Autodesk Inventor part; units mm, degrees
ref_plane "YZ Plane" through (0, 0, 0) normal (1, 0, 0) x (0, 1, 0)
ref_plane "XZ Plane" through (0, 0, 0) normal (0, 1, 0) x (-1, 0, 0)
ref_plane "XY Plane" through (0, 0, 0) normal (0, 0, 1) x (1, 0, 0)
sketch "Sketch1" plane through (0, 0, 0) normal (0, 0, 1) x (1, 0, 0)
  line L0 (-40, -28.4) -> (40, -28.4)
  line L1 (40, -28.4) -> (40, 28.4)
  line L2 (40, 28.4) -> (-40, 28.4)
  line L3 (-40, 28.4) -> (-40, -28.4)
  line L4 (-40, -28.4) -> (40, 28.4) construction
  line L5 (40, -28.4) -> (-40, 28.4) construction
  line L6 (-32.5, -20.9) -> (32.5, -20.9) construction
  line L7 (32.5, -20.9) -> (32.5, 20.9) construction
  line L8 (32.5, 20.9) -> (-32.5, 20.9) construction
  line L9 (-32.5, 20.9) -> (-32.5, -20.9) construction
  line L10 (-32.5, -20.9) -> (32.5, 20.9) construction
  line L11 (32.5, -20.9) -> (-32.5, 20.9) construction
  circle A0 centre (-32.5, -20.9) radius 3.25 construction
  circle A1 centre (32.5, 20.9) radius 3.25 construction
  circle A2 centre (32.5, -20.9) radius 3.25 construction
  line L12 (-40, -13.4) -> (-27.8, -13.4)
  line L13 (-27.8, -13.4) -> (-27.8, 28.4)
  circle A3 centre (-20.3, 20.9) radius 3.25 construction
  line L14 (40, 28.4) -> (32.5, 20.9)
  line L15 (-27.8, 28.4) -> (-20.3, 20.9) construction
  point P0 (0, 0)
  point P1 (34.5, 22.9)
  point P2 (-22.3, 22.9)
  dimension "d0" = 80
  dimension "d1" = 56.8
  dimension "d2" = 41.8
  dimension "d3" = 65
  dimension "d4" = 6.5
  dimension "d5" = 6.5
  dimension "d6" = 6.5
  dimension "d8" = 7.5
  dimension "d9" = 7.5
  dimension "d10" = 7.5
  dimension "d11" = 12.2
  dimension "d12" = 6.5
  dimension "d13" = 7.5
  dimension "d61" = 5.5
  dimension "d62" = 5.5
extrude "Base" add sketch "Sketch1" against normal blind 5.5 contours L3 L12 L13 L2 L1 L0
hole "Mounting Holes" at (32.5, -20.9, 0) at (-32.5, -20.9, 0) at (34.5, 22.9, 0) at (-22.3, 22.9, 0) direction (0, 0, -1) diameter 3.4 end through all
fillet "Fillet1" radius 5 6 edges at (-40, -28.4, -2.75) (-40, -13.4, -2.75) (-27.8, -13.4, -2.75) (-27.8, 28.4, -2.75) (40, 28.4, -2.75) (40, -28.4, -2.75)
sketch "Sketch2" plane through (0, 0, 0) normal (0, 0, 1) x (1, 0, 0)
  circle A0 centre (32.5, -20.9) radius 1.7
  point P0 (0, 0)
  point P1 (6.1, -6.4)
  point P2 (6.1, 11.6)
  dimension "d24" = 6.1
  dimension "d26" = 18
  dimension "d63" = 14.5
hole "Bearing Bore" at (6.1, 11.6, 0) direction (0, 0, -1) diameter 15 end through all counterbore diameter 16.4 counterbore depth 5
sketch "Sketch8" plane through (0, 0, 0) normal (0, 0, 1) x (1, 0, 0)
  line L0 (27.8, 17.4) -> (40, 17.4)
  line L1 (40, 17.4) -> (40, -13.4)
  line L2 (40, -13.4) -> (27.8, -13.4)
  line L3 (27.8, -13.4) -> (27.8, 17.4)
  line L4 (27.8, 17.4) -> (40, -13.4) construction
  line L5 (40, 17.4) -> (27.8, -13.4) construction
  circle A0 centre (34.5, 22.9) radius 1.7
  circle A1 centre (32.5, -20.9) radius 1.7
  line L6 (40, -23.4) -> (40, 23.4)
  line L7 (-35, -28.4) -> (35, -28.4)
  point P0 (0, 0)
  point P1 (33.9, 2)
  dimension "d73" = 12.2
  dimension "d77" = 15
  dimension "d78" = 7.5
  dimension "d79" = 5.5
extrude "Clamp Clearance" cut sketch "Sketch8" against normal blind 10 contours L0 L1 L2 L3
fillet "Fillet3" radius 5 2 edges at (40, 17.4, -2.75) (40, -13.4, -2.75)
sketch "Sketch9" plane through (0, 0, -5.5) normal (0, 0, -1) x (-1, 0, 0)
  circle A0 centre (-34.5, 22.9) radius 1.7
  arc A1 (-32.5, 33) -> (-22.5, 35.5) centre (-32.5, 54.25) ccw construction
  arc A2 (-32.5, 27) -> (-19.6765, 30.2059) centre (-32.5, 54.25) ccw
  arc A3 (-32.5, 39) -> (-25.3235, 40.7941) centre (-32.5, 54.25) ccw
  arc A4 (-32.5, 39) -> (-32.5, 27) centre (-32.5, 33) ccw
  arc A5 (-19.6765, 30.2059) -> (-25.3235, 40.7941) centre (-22.5, 35.5) ccw
  circle A6 centre (-32.5, -31) radius 6
  circle A7 centre (32.5, -31) radius 6
  circle A8 centre (-32.5, -20.9) radius 1.7
  circle A9 centre (32.5, -20.9) radius 1.7
  point P0 (0, 0)
  dimension "d80" = 2
  dimension "d81" = 10.1
  dimension "d82" = 6
  dimension "d83" = 10
  dimension "d84" = 2.5
  dimension "d85" = 15.25
  dimension "d86" = 10.1
  dimension "d87" = 10.1
  dimension "d88" = 12
extrude "Bolt Clearance" cut sketch "Sketch9" against normal blind 10 contours A4 A3 A5 A2 | A6 | A7
sketch "Sketch10" plane through (0, 0, -5.5) normal (0, 0, -1) x (-1, 0, 0)
  line L0 (-27.0926, -28.4) -> (27.0926, -28.4)
  circle A0 centre (-6.1, 11.6) radius 7.5
  point P0 (0, 0)
  point P1 (-15, -22.2)
  point P2 (12, -22.2)
  dimension "d91" = 6.2
  dimension "d92" = 6.2
  dimension "d102" = 15
  dimension "d103" = 12
hole "Lower Block Holes" at (15, -22.2, -5.5) at (-12, -22.2, -5.5) direction (0, 0, 1) diameter 3.4 end through all counterbore diameter 6.5 counterbore depth 3
sketch "Sketch11" plane through (15, -22.2, -2.5) normal (0, 0, -1) x (-1, 0, 0)
  circle A0 centre (0, 0) radius 1.7
  circle A1 centre (27, 0) radius 1.7
  point P0 (15, 22.2)
extrude "Print Feature" add sketch "Sketch11" against normal blind 1
fillet "Fillet4" radius 5 2 edges at (27.8, -13.4, -2.75) (27.8, 17.4, -2.75)
equation "\"d13\" = d10"
properties part number "Extruder Mount Plate 2" material "ABS Plastic"
Build history of the part. All positions in model axes, mm. A direction names the side the tool comes from. Coordinates: 2 decimals unless noted, no trailing zeros. Write each loop counter-clockwise with the first axis right and the second up, starting at its lowest first coordinate (ties: lowest second). Pieces come first, ordered by that corner, then holes.
(1) 3-axis set-ups, long thin cutter, end or side, ignore diameter. For faces 5 (the flat face through (13, 8, -5)), 6 (the flat face through (-1, 0, -5.5)), 7 (the cylindrical face through (38.57, 18.9, -2.79)), 8 (the flat face through (-12, -22, -2.5)): which of +Z, -Z, +X, -X, +Y, -Y reach the whole face in a straight line?
(2) Cut at B-B on y = -1. List the corners of the cut face in (x, z), and give its area (3 significant figures).
(3) Mould opens along Y. For faces 1 (the cylindrical face through (34.47, 27.333, -2.788)), 2 (the cylindrical face through (29.23, 15.9, -2.79)), 3 (the flat face through (-40, -21, -3)), 4 (the flat face through (15, -22, -2.5)) say: pulls with the +Y half, pulls with the -Y half, needs draft (parallel to the pull), parting line crosses it, or undercut.
(4) Drill centre lines: line 1 (Y direction, x = 32.5, z = -3.4); line 2 (X direction, y = 22.9, z = -2.7); line 3 (X direction, y = -22.2, z = -1.1). Where is each one in solid material? Low to high.
(5) Cut at A-A on y = 11.6. List the corners of the cut face in (x, z), and give its area (3 significant figures).
(6) Pin check, flat tips, straight feed: pin 1 Ø1.1 at (x, z) = (34, -3.5) entering from -Y; pin 2 Ø1.8 at (x, z) = (34, -2) entering from +Y; pin 3 Ø1 at (x, y) = (-12, -22.5) entering from +Z; pin 4 Ø4 at (x, y) = (-22.3, 22.9) entering from -Z. Stop position of each tip, or through.
Working result:
1. face 5: +Z
1. face 6: -Z, +X, -X, +Y, -Y
1. face 7: +Z, -Z, +X
1. face 8: -Z
2. outline: (-27.8, -5.5) - (27.8, -5.5) - (27.8, 0) - (-27.8, 0) - close
2. area: 306 mm2
3. face 1: pulls with the +Y half
3. face 2: undercut
3. face 3: needs draft
3. face 4: undercut
4. line 1: y = -25 to -22.6, -19.2 to -13.39, 17.39 to 27
4. line 2: x = -27.8 to -24, -20.6 to 32.8, 36.2 to 40
4. line 3: x = -40 to -33.6, -31.4 to -13.7, -10.3 to 13.3, 16.7 to 31.4, 33.6 to 40
5. outline: (-27.8, -5.5) - (-1.4, -5.5) - (-1.4, -5) - (-2.1, -5) - (-2.1, 0) - (-27.8, 0) - close; (13.6, -5.5) - (27.8, -5.5) - (27.8, 0) - (14.3, 0) - (14.3, -5) - (13.6, -5) - close
5. area: 216 mm2
6. pin 1: stops at y = -25.36
6. pin 2: stops at y = 27.5
6. pin 3: stops at z = -1.5
6. pin 4: stops at z = -5.5
